Geometry check sheet. Reference: the model listing, model coordinates, mm. Face numbers are marked on the shaded views. A direction names the side the tool comes from. Coordinates: 2 decimals unless noted, no trailing zeros. Write each loop counter-clockwise with the first axis right and the second up, starting at its lowest first coordinate (ties: lowest second). Pieces come first, ordered by that corner, then holes. Notation, with made-up numbers: (85, 41) -> (134, 41) arc R17 cw to (134, 70) -> close; hole circle Ø8 at (22, -28). An arc over 180 degrees is marked (long way). Answer as CSV lines item,"result".
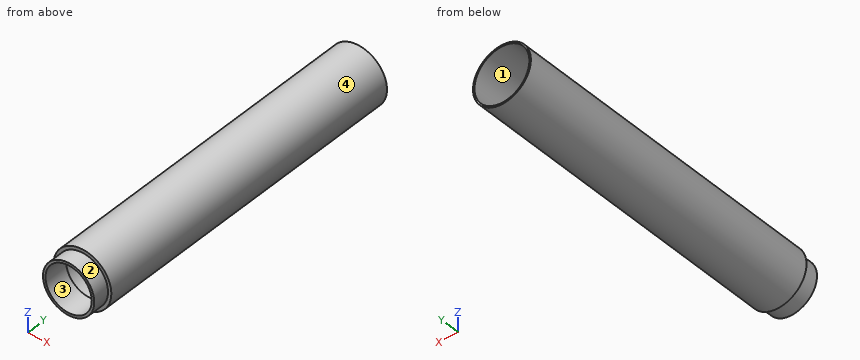
```python
from build123d import *

# Parameters (mm, degrees)
SKETCH1_R           = 15.5
SKETCH1_R_2         = 14
BOSS_EXTRUDE1_DEPTH = 10
SKETCH4_R           = 17.5
SKETCH4_R_2         = 14
BOSS_EXTRUDE2_DEPTH = 200
SKETCH5_R           = 16.6
CUT_EXTRUDE2_DEPTH  = 195


with BuildPart() as part:
    # Sketch1 → Boss-Extrude1 (new body)
    with BuildSketch(Plane(origin=(0, 0, 0), x_dir=(1, 0, 0), z_dir=(0, 1, 0))):
        with Locations(Location((0, 0, 0), (0, 0, 270))):
            Circle(SKETCH1_R)
        with Locations(Location((0, 0, 0), (0, 0, 270))):
            Circle(SKETCH1_R_2, mode=Mode.SUBTRACT)
    extrude(amount=BOSS_EXTRUDE1_DEPTH)

    # Sketch4 → Boss-Extrude2 (add)
    with BuildSketch(Plane(origin=(0, 10, 0), x_dir=(1, 0, 0), z_dir=(0, 1, 0))):
        with Locations(Location((0, 0, 0), (0, 0, 270))):
            Circle(SKETCH4_R)
        with Locations(Location((0, 0, 0), (0, 0, 270))):
            Circle(SKETCH4_R_2, mode=Mode.SUBTRACT)
    extrude(amount=BOSS_EXTRUDE2_DEPTH)

    # Sketch5 → Cut-Extrude2 (cut)
    with BuildSketch(Plane(origin=(0, 210, 0), x_dir=(1, 0, 0), z_dir=(0, 1, 0))):
        with Locations(Location((0, 0, 0), (0, 0, 270))):
            Circle(SKETCH5_R)
    extrude(amount=-CUT_EXTRUDE2_DEPTH, mode=Mode.SUBTRACT)


solid = part.part
```
Item 1: Cross-section at B-B, the plane z = -12. Record the cut outline in (x, y).
Responses:
outline,"(-12.74, 10) -> (-9.81, 10) -> (-9.81, 0) -> (-7.21, 0) -> (-7.21, 15) -> (-11.47, 15) -> (-11.47, 210) -> (-12.74, 210) -> close; (7.21, 0) -> (9.81, 0) -> (9.81, 10) -> (12.74, 10) -> (12.74, 210) -> (11.47, 210) -> (11.47, 15) -> (7.21, 15) -> close"
Item 2: Depth check by flat-ended pin: pin 1 Ø10.5 at (x, z) = (0, -5) entering from -Y; pin 2 Ø5 at (x, y) = (7, 159) entering from -Z; pin 3 Ø3 at (y, z) = (103.5, 4) entering from -X; pin 4 Ø8 at (x, y) = (-6.5, 42) entering from +Z. Enter the tip coordinate at first touch or a pass-through.
Responses:
pin 1,"passes through"
pin 2,"stops at z = -16.91"
pin 3,"stops at x = -17.32"
pin 4,"stops at z = 17.32"
Item 3: Set-up check for the marked faces 1 and 2: record each of +Z, -Z, +X, -X, +Y, -Y from which the full face is reachable in a straight line by a thin tool's end or side.
Responses:
face 1,"+Y"
face 2,"-Y"
Item 4: Cross-section at A-A, the plane x = 0. Record the cut outline in (y, z), plus the area to 3 significant figures.
Responses:
outline,"(0, -15.5) -> (10, -15.5) -> (10, -17.5) -> (210, -17.5) -> (210, -16.6) -> (15, -16.6) -> (15, -14) -> (0, -14) -> close; (0, 14) -> (15, 14) -> (15, 16.6) -> (210, 16.6) -> (210, 17.5) -> (10, 17.5) -> (10, 15.5) -> (0, 15.5) -> close"
area,"416 mm2"
Item 5: Cross-section at C-C, the plane y = 135. Record the cut outline in (x, z).
Responses:
outline,"circle Ø35 at (0, 0); hole circle Ø33.2 at (0, 0)"
Item 6: Thickness scan on probe 1 along X at (y, z) = (196.5, -1); probe 2 along Y at (x, z) = (10, 12); probe 3 along X at (y, z) = (8.75, 0). Record the ranges inside material, lowest first.
Responses:
probe 1,"x = -17.47 to -16.57, 16.57 to 17.47"
probe 2,"y = 10 to 15"
probe 3,"x = -15.5 to -14, 14 to 15.5"
Item 7: Release check for a two-part mould opening along Z. For the marked faces 3 and 4 record: +Z half, -Z half, draft (parallel to the pull), parting line (faces both ways), or undercut.
Responses:
face 3,"undercut"
face 4,"parting line"
